Autodesk Fusion 360 part; units mm, degrees
sketch "top" plane through (0, 0, 0) normal (0, 1, 0) x (1, 0, 0)
  line L0 (2.75, -2.75) -> (-2.75, -2.75)
  line L1 (-2.75, -2.75) -> (-2.75, 2.75)
  line L2 (-2.75, 2.75) -> (2.75, 2.75)
  line L3 (2.75, 2.75) -> (2.75, -2.75)
  line L4 (2.75, -2.75) -> (-2.75, 2.75) construction
  line L5 (-2.75, -2.75) -> (2.75, 2.75) construction
  line L6 (-51.8482, 4.55) -> (53.2802, 4.55)
  line L7 (10, -10) -> (-10, -10)
  line L8 (-10, -10) -> (-10, 10)
  line L9 (-10, 10) -> (10, 10)
  line L10 (10, 10) -> (10, -10)
  line L11 (10, -10) -> (-10, 10) construction
  line L12 (-10, -10) -> (10, 10) construction
  line L13 (2.75, 2.75) -> (2.75, 4.55)
  line L14 (-2.75, 2.75) -> (-2.75, 4.55)
  dimension "d1" = 5.5
  dimension "d2" = 5.5
  dimension "d3" = 1.8
  dimension "d4" = 20
  dimension "d5" = 20
extrude "Extrude1" add sketch "top" along normal blind 3 contours L0 L1 L3 L6 L7 L8 L10 L13 L14 | L2 L6 L13 L14
sketch "hole" plane through (0, 0, 0) normal (0, 0, 1) x (1, 0, 0)
  line L0 (0, 0) -> (0, 32.5783)
  circle A0 centre (0, 8.4) radius 8
  line L1 (0, 0.4) -> (15.5935, 0.4) construction
  line L2 (-10, 0) -> (10, 0) construction
  line L3 (10, 0) -> (10, 3) construction
  line L4 (10, 3) -> (-10, 3) construction
  line L5 (-10, 3) -> (-10, 0) construction
  line L6 (5.9025, 3) -> (10, 3)
  line L7 (5.9025, 3) -> (14.475, 0.4)
  line L8 (10, 3) -> (14.475, 3)
  line L9 (14.475, 3) -> (14.475, 0.4)
  point P0 (0, 0.4)
  point P1 (10, 0.4)
  dimension "d8" = 16
  dimension "d9" = 0.4
revolve "Revolve1" cut sketch "hole" angle 360 about axis through (0, 0, 0) along (0, 1, 0) contours L6 L7 L8 L9 | L0 A0 picked at (2.6374, 8.0063)
fillet "Fillet1" radius 2 4 edges at (10, 0.2505, 10) (-10, 0.2505, 10) (-10, 0.729, -4.55) (10, 0.729, -4.55)
sketch "sticky" plane through (0, 0, 0) normal (0, 1, 0) x (1, 0, 0)
  arc A0 (10, 2.55) -> (8, 4.55) centre (8, 2.55) ccw
  line L0 (10, 2.55) -> (10, -8)
  arc A1 (8, -10) -> (10, -8) centre (8, -8) ccw
  line L1 (8, -10) -> (-8, -10)
  arc A2 (-10, -8) -> (-8, -10) centre (-8, -8) ccw
  line L2 (-10, -8) -> (-10, 2.55)
  arc A3 (-8, 4.55) -> (-10, 2.55) centre (-8, 2.55) ccw
  line L3 (-8, 4.55) -> (8, 4.55)
  line L4 (2.75, 2.75) -> (-2.75, 2.75)
  line L5 (-2.75, 2.75) -> (-2.75, -2.75)
  line L6 (-2.75, -2.75) -> (2.75, -2.75)
  line L7 (2.75, -2.75) -> (2.75, 2.75)
Read the model definition and answer for the solid it produces. Units are mm, in the model's axes. A direction names the side the tool comes from. Coordinates: 2 decimals unless noted, no trailing zeros. Order: outer loops, then holes, each group sorted by start corner. A loop starts at its lowest first (then second) coordinate and runs counter-clockwise, first axis right, second up. Notation, with made-up numbers: (50.5, 34.25) - (97.5, 34.25) arc R27 cw to (97.5, 60.25) - close; hole circle Ø10 at (-6, 56). An arc over 180 degrees is marked (long way). Answer as a JSON object with one key per item and string values. Group by question number.
Item 1: Consider probe 1 along X at (y, z) = (0.9, -1); probe 2 along Z at (x, y) = (-1.5, 0.35); probe 3 along Y at (x, z) = (-6, -3.25). Determine where each line is inside the solid, lowest interval first. Write a range as from..to.
Item 2: Section D-D (y = 2.45) is taken. Give the vertices of the cut face in (x, z).
Item 3: A tool of negligible diameter and unlimited length cuts with its end or side. For faces 4 (the face through (0, 0.5, -2.75)), 5 (the face through (0.22, 2.86, 6.36)), from which of +Z, -Z, +X, -X, +Y, -Y can it reach the whole face along a straight path? Write none if from no direction.
Item 4: The mould has two halves that part along X. Classify faces 1 (the face through (10, 1, 3)), 2 (the face through (2.75, 0.5, 0)), 3 (the face through (0, 1, 10)): +X half, -X half, draft (parallel to the pull), parting line (faces both ways), or undercut.
Item 5: Section B-B (y = 0.5) is taken. Give the vertices of the cut face in (x, z).
Item 6: Section A-A (z = 0) is taken. Give the vertices of the cut face in (x, y).
Item 7: Section C-C (x = 0) is taken. Give the vertices of the cut face in (y, z).
Results are:
{
 "1": {"probe 1": "x = -10..-2.75, 2.75..10", "probe 2": "z = -4.55..-2.75, 2.75..10", "probe 3": "y = 0..2.72"},
 "2": {"outline": "(-6.23, -4.55) - (-2.81, -4.55) arc R5.35 cw (long way) to (2.81, -4.55) - (6.23, -4.55) arc R7.72 ccw (long way) to start"},
 "3": {"face 4": "+Y, -Y", "face 5": "+Y"},
 "4": {"face 1": "+X half", "face 2": "undercut", "face 3": "draft"},
 "5": {"outline": "(-10, -2.55) arc R2 ccw to (-8, -4.55) - (8, -4.55) arc R2 ccw to (10, -2.55) - (10, 8) arc R2 ccw to (8, 10) - (-8, 10) arc R2 ccw to (-10, 8) - close; hole (-2.75, -2.75) - (2.75, -2.75) - (2.75, 2.75) - (-2.75, 2.75) - close"},
 "6": {"outline": "(-10, 0) - (-2.75, 0) - (-2.75, 0.89) arc R8 cw to (-5.9, 3) - (-10, 1.76) - close; (2.75, 0) - (10, 0) - (10, 1.76) - (5.9, 3) arc R8 cw to (2.75, 0.89) - close"},
 "7": {"outline": "(0, -4.55) - (1.82, -4.55) arc R8 cw to (0.89, -2.75) - (0, -2.75) - close; (0, 2.75) - (0.89, 2.75) arc R8 cw to (3, 5.9) - (1.76, 10) - (0, 10) - close"}
}
